from build123d import *

# Parameters (mm, degrees)
SKETCH_1_R               = 49
EXTRUDE_1_DEPTH          = 3
CUT_EXTRUDE_3_DEPTH      = 4
CUT_EXTRUDE_4_DEPTH      = 4
PATTERN_CIRCULAR_4_COUNT = 2
SKETCH_2_R               = 1.25
CUT_EXTRUDE_5_DEPTH      = 4
PATTERN_CIRCULAR_5_COUNT = 4
PATTERN_CIRCULAR_6_COUNT = 4


with BuildPart() as part:
    # 草图1 → 凸台-拉伸1 (new body)
    with BuildSketch(Plane(origin=(0, 0, 0), x_dir=(1, 0, 0), z_dir=(0, 1, 0))):
        Circle(SKETCH_1_R)
    extrude(amount=EXTRUDE_1_DEPTH)

    # 草图5 → 切除-拉伸3 (cut, through all)
    with BuildSketch(Plane(origin=(0, 3, 0), x_dir=(1, 0, 0), z_dir=(0, 1, 0))):
        with BuildLine():
            Line((7, 42.420036355), (7, 7))
            Line((7, 7), (42.420036355, 7))
            ThreePointArc((42.420036355, 7), (30.401147054, 30.401147054), (7, 42.420036355))
        make_face()
    cut_extrude_3 = extrude(amount=-CUT_EXTRUDE_3_DEPTH, mode=Mode.SUBTRACT)

    # 草图6 → 切除-拉伸4 (cut, through all)
    with BuildSketch(Plane(origin=(0, 3, 0), x_dir=(1, 0, 0), z_dir=(0, 1, 0))):
        with BuildLine():
            Line((-12.3, -1.5), (-37.3, -1.5))
            ThreePointArc((-37.3, -1.5), (-38.8, 0), (-37.3, 1.5))
            Line((-37.3, 1.5), (-12.3, 1.5))
            ThreePointArc((-12.3, 1.5), (-10.8, 0), (-12.3, -1.5))
        make_face()
    cut_extrude_4 = extrude(amount=-CUT_EXTRUDE_4_DEPTH, mode=Mode.SUBTRACT)

    # 阵列(圆周)4: 切除-拉伸4 ×2 about axis
    pattern_circular_4_axis = Axis((0, 0, 0), (0, 1, 0))
    for i in range(1, PATTERN_CIRCULAR_4_COUNT):
        add(cut_extrude_4.rotate(pattern_circular_4_axis, i * 360 / PATTERN_CIRCULAR_4_COUNT), mode=Mode.SUBTRACT)

    # 草图2 → 切除-拉伸5 (cut, through all)
    with BuildSketch(Plane(origin=(0, 3, 0), x_dir=(1, 0, 0), z_dir=(0, 1, 0))):
        with Locations((0, 46.1)):
            Circle(SKETCH_2_R)
    cut_extrude_5 = extrude(amount=-CUT_EXTRUDE_5_DEPTH, mode=Mode.SUBTRACT)

    # 阵列(圆周)5: 切除-拉伸5 ×4 about axis
    pattern_circular_5_axis = Axis((0, 0, 0), (0, 1, 0))
    for i in range(1, PATTERN_CIRCULAR_5_COUNT):
        add(cut_extrude_5.rotate(pattern_circular_5_axis, i * 360 / PATTERN_CIRCULAR_5_COUNT), mode=Mode.SUBTRACT)

    # 阵列(圆周)6: 切除-拉伸3 ×4 about axis
    pattern_circular_6_axis = Axis((0, 0, 0), (0, 1, 0))
    for i in range(1, PATTERN_CIRCULAR_6_COUNT):
        add(cut_extrude_3.rotate(pattern_circular_6_axis, i * 360 / PATTERN_CIRCULAR_6_COUNT), mode=Mode.SUBTRACT)


solid = part.part
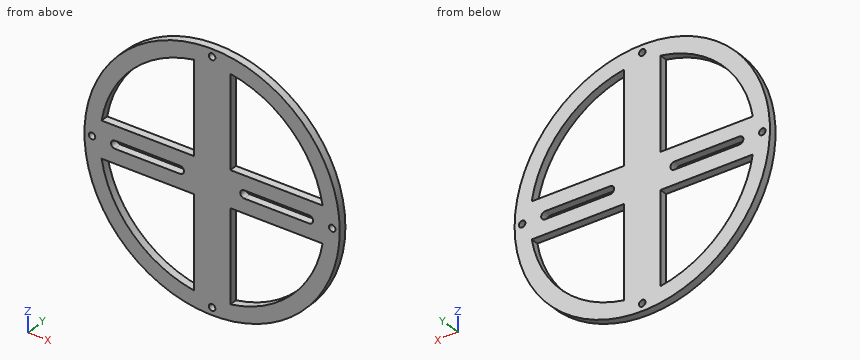
Design review of the part built by this model. Coordinates are the model's own, in mm. Give positions to 0.01 mm unless a question says otherwise; leave off trailing zeros. Loops run counter-clockwise (first coordinate to the right, second up) from the corner with the lowest first, then second, coordinate; pieces in that order, holes last. Notation, with made-up numbers: M -31,56 L 8,56 A33 ccw 8,95 Z; hole C -15.5,67 d5. An arc over 180 degrees is marked long. One line per question, with ' | ' between items. Start each with the question number.
1. Add section A-A (x = 0). Write out the cut boundary in (y, z), plus the area to 3 significant figures.
2. Add section B-B (z = 0). Write out the cut boundary in (x, y).
3. Add section C-C (z = 46.1). Write out the cut boundary in (x, y), plus the area to 3 significant figures.
4. Insertion check: P1, Ø0.9, axis at y = 1, z = -30.5, coming from the +X side; P2, Ø0.9, axis at x = 20.5, y = 1.5, coming from the -Z side; P3, Ø0.9, axis at y = 2, z = 28.5, coming from the +X side. Each pin has a flat end and moves straight along its axis. Give the tip position at first contact, or say it passes through.
5. To check wall thickness, follow L1, parallel to X at y = 2.2, z = 0; L2, parallel to Z at x = 0, y = 1.7; L3, parallel to X at y = 0.45, z = 37. State the ranges of each line that lie inside material, in increasing order.
6. Add section D-D (y = 2.5). Give the number of separate pieces and of enclosed holes in the cut face, plus the area to 3 significant figures.
Worked out:
1) outline: M 0,-49 L 3,-49 L 3,-47.35 L 0,-47.35 Z; M 0,-44.85 L 3,-44.85 L 3,44.85 L 0,44.85 Z; M 0,47.35 L 3,47.35 L 3,49 L 0,49 Z | area: 279 mm²
2) outline: M -49,0 L -47.35,0 L -47.35,3 L -49,3 Z; M -44.85,0 L -38.8,0 L -38.8,3 L -44.85,3 Z; M -10.8,0 L 10.8,0 L 10.8,3 L -10.8,3 Z; M 38.8,0 L 44.85,0 L 44.85,3 L 38.8,3 Z; M 47.35,0 L 49,0 L 49,3 L 47.35,3 Z
3) outline: M -16.61,0 L -1.25,0 L -1.25,3 L -16.61,3 Z; M 1.25,0 L 16.61,0 L 16.61,3 L 1.25,3 Z | area: 92.1 mm²
4) P1: stops at x = 38.7 | P2: stops at z = -44.71 | P3: stops at x = 40.18
5) L1: x = -49 to -47.35, -44.85 to -38.8, -10.8 to 10.8, 38.8 to 44.85, 47.35 to 49 | L2: z = -49 to -47.35, -44.85 to 44.85, 47.35 to 49 | L3: x = -32.12 to -21.9, -7 to 7, 21.9 to 32.12
6) separate pieces: 1 | enclosed holes: 10 | area: 3,750 mm²
